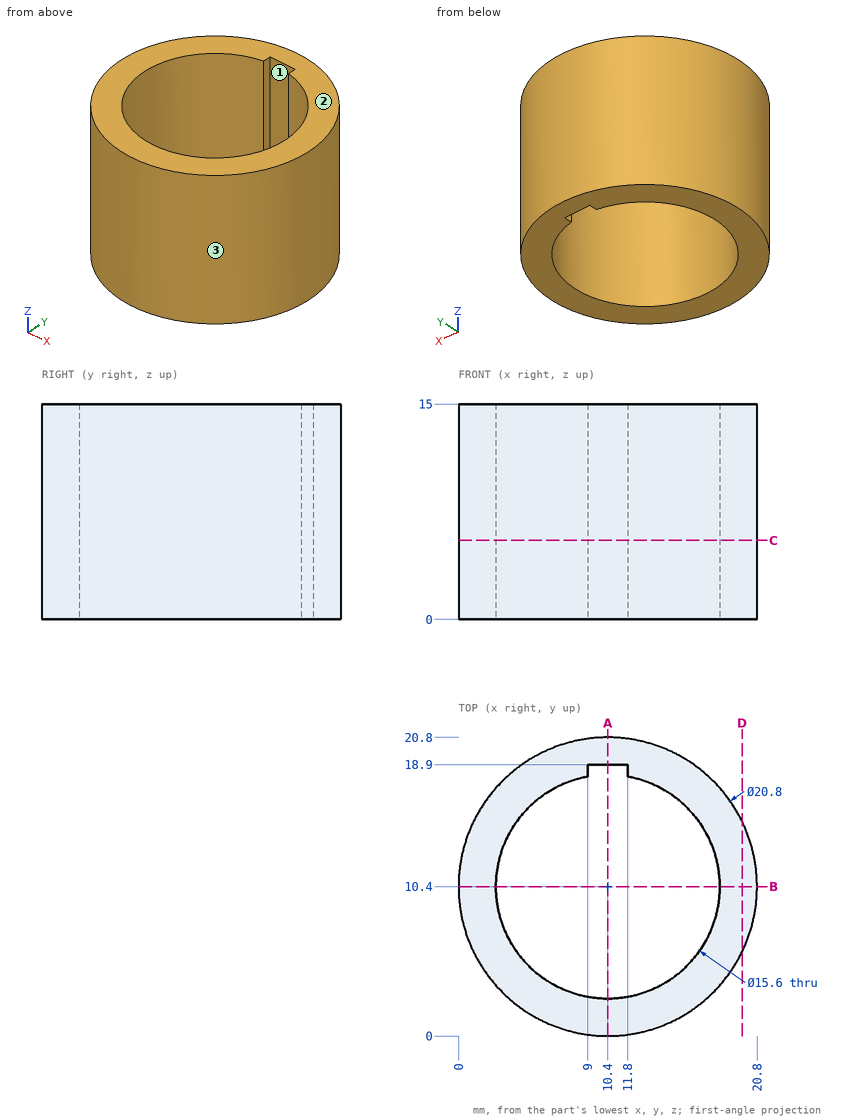
The figure shows three views and two pictorial views of one solid part (mm, origin at its lowest corner). Answer the questions. Give positions to 0.01 mm unless a question says otherwise; leave off trailing zeros. Write each loop counter-clockwise with the first axis right and the second up, starting at its lowest first coordinate (ties: lowest second). Pieces come first, ordered by that corner, then holes.
Q1. The part is cut by section A-A on x = 10.4. Give the vertices of the cut face in (y, z), and give its area (3 significant figures).
Answer:
outline: (0, 0) - (2.6, 0) - (2.6, 15) - (0, 15) - close; (18.9, 0) - (20.8, 0) - (20.8, 15) - (18.9, 15) - close
area: 67.5 mm2
Q2. For a pull along Y with two mould halves and no side action, classify the marked faces 1, 2 and 3 as released by +Y, released by -Y, zero draft, split by the parting line, or undercut.
Answer:
face 1: undercut
face 2: zero draft
face 3: split by the parting line
Q3. The part is cut by section D-D on x = 19.75. Give the vertices of the cut face in (y, z).
Answer:
outline: (5.85, 0) - (14.95, 0) - (14.95, 15) - (5.85, 15) - close
Q4. Given pin 1 (0.8 mm diameter, centred on x = 11, z = 9, fed in from -Y); pin 2 (0.9 mm diameter, centred on y = 18.5, z = 10.5, fed in from -X), each flat-ended and moving along its own axis, determine where each tip first touches the part or whether it passes through.
Answer:
pin 1: stops at y = 0
pin 2: stops at x = 3.35
Q5. Straight lines are drawn through the part: L1, parallel to Y at x = 10.4, z = 6.5; L2, parallel to Y at x = 4.5, z = 6.75; L3, parallel to X at y = 14.25, z = 11. For each, find the intervals that lie inside material, in ascending order.
Answer:
L1: y = 0 to 2.6, 18.9 to 20.8
L2: y = 1.84 to 5.3, 15.5 to 18.96
L3: x = 0.74 to 3.62, 17.18 to 20.06
Q6. The part is cut by section C-C on z = 5.5. Give the vertices of the cut face in (x, y).
Answer:
outline: circle Ø20.8 at (10.4, 10.4); hole (9, 18.07) arc R7.8 ccw (long way) to (11.8, 18.07) - (11.8, 18.9) - (9, 18.9) - close
Q7. The part is cut by section B-B on y = 10.4. Give the vertices of the cut face in (x, z), and give its area (3 significant figures).
Answer:
outline: (0, 0) - (2.6, 0) - (2.6, 15) - (0, 15) - close; (18.2, 0) - (20.8, 0) - (20.8, 15) - (18.2, 15) - close
area: 78.0 mm2
